Drawing for the job (mm, zero at the part's lowest x, y, z). Round coordinates to 2 decimals unless told otherwise and drop trailing zeros. Write each loop counter-clockwise with the first axis right and the second up, starting at its lowest first coordinate (ties: lowest second). Pieces come first, ordered by that corner, then holes. Notation, with made-up numbers: (-14, 78.5) -> (37, 78.5) arc R18 cw to (37, 90.5) -> close; hole circle Ø6 at (-22, 38). An arc over 180 degrees is marked (long way). Answer in a Markdown table with one row per item. Add a question column.
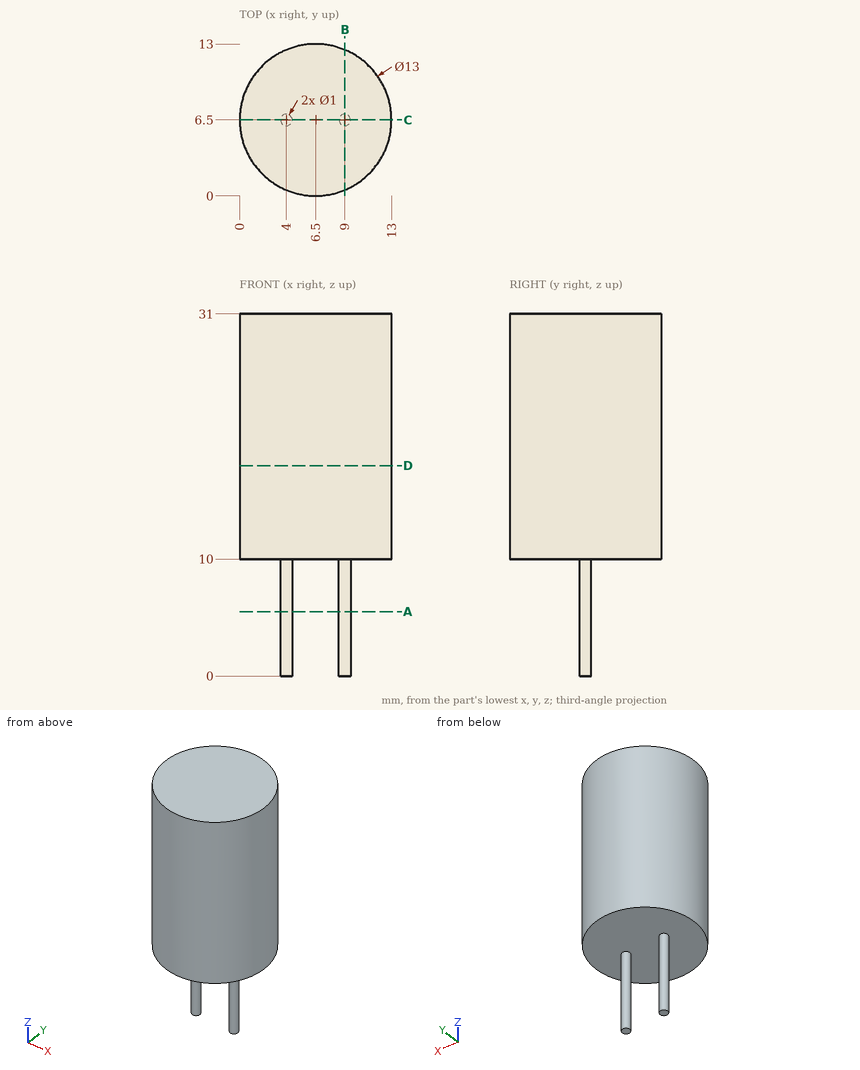
(1) Saw through at C-C (y = 6.5). List the corners of the cut face in (x, z).
(2) Saw through at A-A (z = 5.5). List the corners of the cut face in (x, y), plus the area to 3 significant figures.
(3) Saw through at B-B (x = 9). List the corners of the cut face in (y, z).
(4) Drop flat-ended pins along their axis: P1, Ø1, axis at y = 5.5, z = 19.5, coming from the -X side; P2, Ø3, axis at x = 1.5, z = 20.5, coming from the +Y side; P3, Ø2, axis at x = 10, y = 10.5, coming from the -Z side. Give the stop position or say it passes through.
(5) Probe line 1 along Z through (x, y) = (8.5, 3.75); line 2 along Y through (x, z) = (2, 14.5); line 3 along Y through (x, z) = (4, 5.5). List the from-to ranges inside material, lowest first.
(6) Saw through at D-D (z = 18). List the corners of the cut face in (x, y), plus the area to 3 significant figures.
Answer sheet:
| question | item | result |
|---|---|---|
| 1 | outline | (0, 10) -> (3.5, 10) -> (3.5, 0) -> (4.5, 0) -> (4.5, 10) -> (8.5, 10) -> (8.5, 0) -> (9.5, 0) -> (9.5, 10) -> (13, 10) -> (13, 31) -> (0, 31) -> close |
| 2 | outline | circle Ø1 at (4, 6.5); circle Ø1 at (9, 6.5) |
| 2 | area | 1.57 mm² |
| 3 | outline | (0.5, 10) -> (6, 10) -> (6, 0) -> (7, 0) -> (7, 10) -> (12.5, 10) -> (12.5, 31) -> (0.5, 31) -> close |
| 4 | P1 | stops at x = 0.02 |
| 4 | P2 | stops at y = 11.98 |
| 4 | P3 | stops at z = 10 |
| 5 | line 1 | z = 10 to 31 |
| 5 | line 2 | y = 1.81 to 11.19 |
| 5 | line 3 | y = 6 to 7 |
| 6 | outline | circle Ø13 at (6.5, 6.5) |
| 6 | area | 133 mm² |
